from build123d import *

# Parameters (mm, degrees)
BOSS_EXTRUDE1_DEPTH = 3.175
SKETCH2_R           = 1.905
CUT_EXTRUDE1_DEPTH  = 9.525
CUT_EXTRUDE2_DEPTH  = 6.35
FILLET1_R           = 2.54
FILLET2_R           = 1.27


with BuildPart() as part:
    # Sketch1 → Boss-Extrude1 (new body, symmetric)
    with BuildSketch(Plane.XY):
        with BuildLine():
            Line((-5.499261314, 3.175), (14.408622788, 37.656466735))
            Line((14.408622788, 37.656466735), (8.909361473, 40.831466735))
            Line((8.909361473, 40.831466735), (-47.625, 50.8))
            Line((-47.625, 50.8), (-47.625, 79.375))
            Line((-47.625, 79.375), (-57.15, 79.375))
            Line((-57.15, 79.375), (-57.15, 37.895014625))
            Line((-57.15, 37.895014625), (8.909361473, -40.831466735))
            Line((8.909361473, -40.831466735), (14.408622788, -37.656466735))
            Line((14.408622788, -37.656466735), (-5.499261314, -3.175))
            ThreePointArc((-5.499261314, -3.175), (-6.35, 0), (-5.499261314, 3.175))
        make_face()
    extrude(amount=BOSS_EXTRUDE1_DEPTH, both=True)

    # Sketch2 → Cut-Extrude1 (cut)
    with BuildSketch(Plane(origin=(-47.625, 0, 0), x_dir=(0, 0, -1), z_dir=(1, 0, 0))):
        with Locations((0, 73.025)):
            Circle(SKETCH2_R)
    extrude(amount=-CUT_EXTRUDE1_DEPTH, mode=Mode.SUBTRACT)

    # Sketch3 → Cut-Extrude2 (cut)
    with BuildSketch(Plane.XY.offset(3.175)):
        Polygon((-47.625, 44.352041015), (-50.337094235, 39.654556005), (-15.642242309, -1.693158423), (5.530597046, 34.97927508), align=None)
    extrude(amount=-CUT_EXTRUDE2_DEPTH, mode=Mode.SUBTRACT)

    # Fillet1
    fillet1_edges = [part.edges().sort_by_distance(p)[0] for p in [
        (-47.625, 50.8, 0),
        (8.909361473, 40.831466735, 0),
        (14.408622788, 37.656466735, 0),
        (14.408622788, -37.656466735, 0),
        (8.909361473, -40.831466735, 0),
        (-57.15, 37.895014625, 0),
        (-47.625, 44.352041015, 0),
        (5.530597046, 34.97927508, 0),
        (-15.642242309, -1.693158423, 0),
        (-50.337094235, 39.654556005, 0),
    ]]
    fillet(fillet1_edges, radius=FILLET1_R)

    # Fillet2
    fillet2_edges = [part.edges().sort_by_distance(p)[0] for p in [
        (-57.15, 79.375, 0),
        (-47.625, 79.375, 0),
    ]]
    fillet(fillet2_edges, radius=FILLET2_R)


solid = part.part
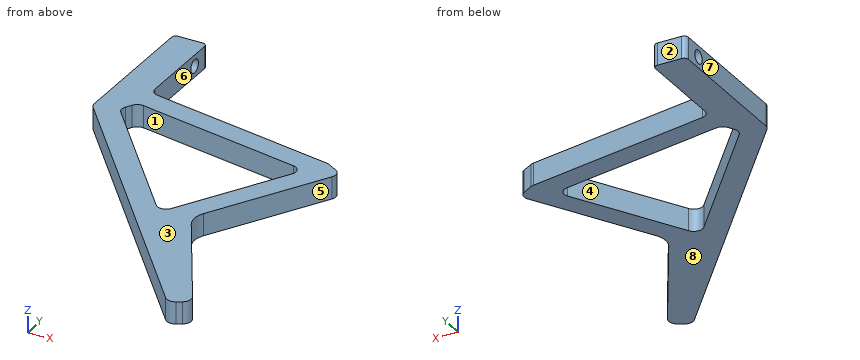
Work out the finished part from the listing and answer in its coordinate system (mm). Face numbers are marked on the shaded views. A direction names the side the tool comes from. Give positions to 0.01 mm unless a question says otherwise; leave off trailing zeros. Loops run counter-clockwise (first coordinate to the right, second up) from the corner with the lowest first, then second, coordinate; pieces in that order, holes last. Notation, with made-up numbers: (79.25, -16) - (123.25, -16) arc R18 ccw to (123.25, 18) - close; hole circle Ø3 at (46, 62.25). An arc over 180 degrees is marked (long way). Answer in a Markdown table with one row per item. Add a question column.
Q1. The part is cut by section C-C (x = 6). Determine the outline of the cut face in (y, z) (3 decimals).
Q2. Determine the mould class of the marked faces 1, 2 and 3 for opening direction Y: released by +Y, released by -Y, zero draft, split by the parting line, or undercut.
Q3. Each of these flat-tipped pins is pushed along its axis until it touches: P1, Ø3, axis at x = -33.5, z = 1, coming from the -Y side; P2, Ø5, axis at x = -40, y = 39.5, coming from the -Z side (3 decimals); P3, Ø3, axis at y = 21, z = -0.5, coming from the -X side. Where does it stop, or does it pass through?
Q4. A tool of negligible diameter and unlimited length cuts with its end or side. For the marked faces 4, 5, 6, 7 and 8, from which of +Z, -Z, +X, -X, +Y, -Y can it reach the whole face along a straight path? Write none if from no direction.
Q5. The part is cut by section D-D (y = 68.5). Determine the outline of the cut face in (x, z) (3 decimals).
Q6. The part is cut by section A-A (z = 0). State how many separate pieces and enclosed holes the cut face has, and give its area (3 significant figures).
Q7. Consider line 1 along Y through (x, z) = (-3, -0.5); line 2 along X through (y, z) = (4.5, 2); line 3 along Y through (x, z) = (-15, -1.5). Determine where each line is inside the solid, lowest interval first.
Q8. The part is cut by section B-B (y = 25). Determine the outline of the cut face in (x, z) (3 decimals).
Solution:
| question | item | result |
|---|---|---|
| 1 | outline | (-37.364, -3.175) - (-23.092, -3.175) - (-23.092, 3.175) - (-37.364, 3.175) - close; (23.092, -3.175) - (41.344, -3.175) - (41.344, 3.175) - (23.092, 3.175) - close |
| 2 | face 1 | undercut |
| 2 | face 2 | released by +Y |
| 2 | face 3 | zero draft |
| 3 | P1 | stops at y = 7.92 |
| 3 | P2 | passes through |
| 3 | P3 | stops at x = -44.23 |
| 4 | face 4 | +Z, -Z |
| 4 | face 5 | +Z, -Z, +X |
| 4 | face 6 | +Z, -Z, +X, +Y |
| 4 | face 7 | +Z, -Z, -X, +Y, -Y |
| 4 | face 8 | -Z, +X, -X, +Y, -Y |
| 5 | outline | (-57.15, -3.175) - (-47.625, -3.175) - (-47.625, 3.175) - (-57.15, 3.175) - close |
| 6 | separate pieces | 2 |
| 6 | enclosed holes | 1 |
| 6 | area | 1,810 mm² |
| 7 | line 1 | y = -26.64 to -7.5, 7.5 to 20.2, 36.48 to 42.93 |
| 7 | line 2 | x = -29.13 to -20.84, -12.07 to -4.73 |
| 7 | line 3 | y = -12.34 to 0.4, 38.6 to 45.05 |
| 8 | outline | (-46.33, -3.175) - (-38.04, -3.175) - (-38.04, 3.175) - (-46.33, 3.175) - close; (-0.231, -3.175) - (7.101, -3.175) - (7.101, 3.175) - (-0.231, 3.175) - close |
